The listing builds one solid part. Answer for the finished solid, in the listing's coordinates (mm). A direction names the side the tool comes from. Give positions to 0.01 mm unless a question says otherwise; leave off trailing zeros. Write each loop counter-clockwise with the first axis right and the second up, starting at its lowest first coordinate (ties: lowest second). Pieces come first, ordered by that corner, then holes. Notation, with made-up numbers: (34, 31.25) -> (87, 31.25) arc R22 ccw to (87, 64.25) -> close; hole circle Ø11 at (12.5, -33). An arc over 180 degrees is marked (long way). Put each result on its own line as item: value. Start each with the question number.
1) For faces 4 (the flat face through (8, -11, 1)), 5 (the flat face through (5.4, -27, 2)), 6 (the flat face through (52, -36, 1)), 7 (the flat face through (14.5, -38, 1)), determine the directions among +Z, -Z, +X, -X, +Y, -Y from which every point of the face is accessible in a straight line to the end or side of a thin tool.
2) For a pull along Y with two mould halves and no side action, classify faces 1 (the flat face through (51, -11, 1)), 2 (the flat face through (29, -22, 1)), 3 (the flat face through (4, -22, 2)) as released by +Y, released by -Y, zero draft, split by the parting line, or undercut.
3) A cutting plane is placed at B-B (y = -31). Write down the section's boundary in (x, z), then the cut area to 3 significant figures.
4) A cutting plane is placed at D-D (y = -4.95). Write down the section's boundary in (x, z), then the cut area to 3 significant figures.
5) Find the intervals of material crossed by line 1 along Y through (x, z) = (54.5, 2.4); line 2 along X through (y, z) = (-23, 2); line 3 along X through (y, z) = (-13, 0.55), in increasing order. Write a range as from..to.
6) A cutting plane is placed at C-C (z = 0.55). Write down the section's boundary in (x, y), then the cut area to 3 significant figures.
7) A cutting plane is placed at A-A (x = 54.5). Write down the section's boundary in (y, z), then the cut area to 3 significant figures.
8) A flat-ended cylindrical pin translates along its axis: pin 1 Ø1.4 at (x, z) = (55, 1) entering from -Y. Find the tip coordinate at first contact, or state that the pin passes through.
from build123d import *

# Parameters (mm, degrees)
SKETCH1_R           = 2.3
BOSS_EXTRUDE1_DEPTH = 3
SKETCH3_W           = 2.8
SKETCH3_H           = 10
CUT_EXTRUDE1_DEPTH  = 10
SKETCH4_W           = 30
SKETCH4_H           = 3
BOSS_EXTRUDE2_DEPTH = 5


with BuildPart() as part:
    # Sketch1 → Boss-Extrude1 (new body)
    with BuildSketch(Plane.XY):
        Polygon((0, 0), (8, 0), (8, -22), (51, -22), (51, 0), (59, 0), (59, -36), (0, -36), align=None)
        with Locations((4.5, -15.05)):
            Circle(SKETCH1_R, mode=Mode.SUBTRACT)
        with Locations((4.5, -4.95)):
            Circle(SKETCH1_R, mode=Mode.SUBTRACT)
        with Locations((54.5, -4.95)):
            Circle(SKETCH1_R, mode=Mode.SUBTRACT)
        with Locations((54.5, -15.05)):
            Circle(SKETCH1_R, mode=Mode.SUBTRACT)
    extrude(amount=BOSS_EXTRUDE1_DEPTH)

    # Sketch3 → Cut-Extrude1 (cut)
    with BuildSketch(Plane.XY.offset(3)):
        with Locations((4, -27)):
            Rectangle(SKETCH3_W, SKETCH3_H)
        with Locations((55, -27)):
            Rectangle(SKETCH3_W, SKETCH3_H)
    extrude(amount=-CUT_EXTRUDE1_DEPTH, mode=Mode.SUBTRACT)

    # Sketch4 → Boss-Extrude2 (add)
    with BuildSketch(Plane.XZ.offset(36)):
        with Locations((29.5, 1.5)):
            Rectangle(SKETCH4_W, SKETCH4_H)
    extrude(amount=BOSS_EXTRUDE2_DEPTH)


solid = part.part
Reply:
1. face 4: +Z, -Z, +Y
1. face 5: +Z, -Z
1. face 6: +Z, -Z, +X, -Y
1. face 7: +Z, -Z, -X, -Y
2. face 1: zero draft
2. face 2: released by +Y
2. face 3: undercut
3. outline: (0, 0) -> (2.6, 0) -> (2.6, 3) -> (0, 3) -> close; (5.4, 0) -> (53.6, 0) -> (53.6, 3) -> (5.4, 3) -> close; (56.4, 0) -> (59, 0) -> (59, 3) -> (56.4, 3) -> close
3. area: 160 mm2
4. outline: (0, 0) -> (2.2, 0) -> (2.2, 3) -> (0, 3) -> close; (6.8, 0) -> (8, 0) -> (8, 3) -> (6.8, 3) -> close; (51, 0) -> (52.2, 0) -> (52.2, 3) -> (51, 3) -> close; (56.8, 0) -> (59, 0) -> (59, 3) -> (56.8, 3) -> close
4. area: 20.4 mm2
5. line 1: y = -36..-32, -22..-17.35, -12.75..-7.25, -2.65..0
5. line 2: x = 0..2.6, 5.4..53.6, 56.4..59
5. line 3: x = 0..3.46, 5.54..8, 51..53.46, 55.54..59
6. outline: (0, -36) -> (14.5, -36) -> (14.5, -41) -> (44.5, -41) -> (44.5, -36) -> (59, -36) -> (59, 0) -> (51, 0) -> (51, -22) -> (8, -22) -> (8, 0) -> (0, 0) -> close; hole circle Ø4.6 at (4.5, -15.05); hole circle Ø4.6 at (4.5, -4.95); hole (2.6, -32) -> (5.4, -32) -> (5.4, -22) -> (2.6, -22) -> close; hole circle Ø4.6 at (54.5, -15.05); hole circle Ø4.6 at (54.5, -4.95); hole (53.6, -32) -> (56.4, -32) -> (56.4, -22) -> (53.6, -22) -> close
6. area: 1,210 mm2
7. outline: (-36, 0) -> (-32, 0) -> (-32, 3) -> (-36, 3) -> close; (-22, 0) -> (-17.35, 0) -> (-17.35, 3) -> (-22, 3) -> close; (-12.75, 0) -> (-7.25, 0) -> (-7.25, 3) -> (-12.75, 3) -> close; (-2.65, 0) -> (0, 0) -> (0, 3) -> (-2.65, 3) -> close
7. area: 50.4 mm2
8. pin 1: stops at y = -36
